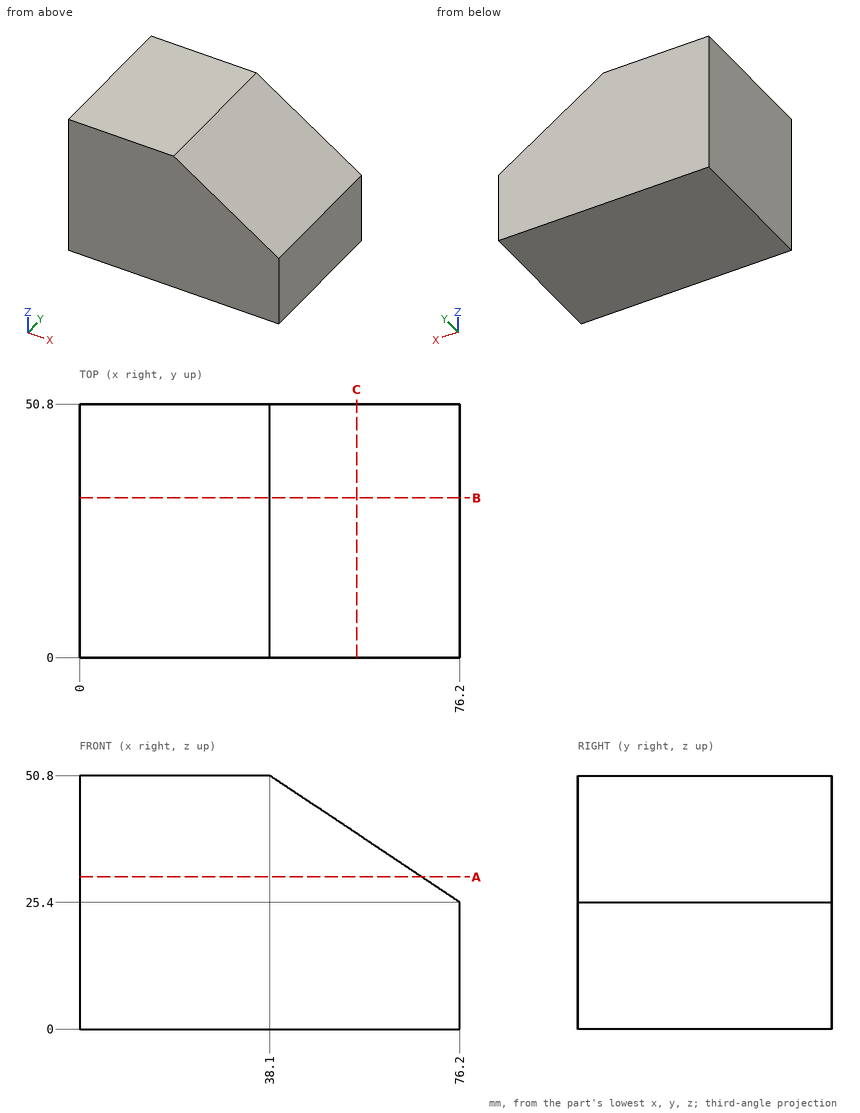
Job drawing, mm, ordinate dimensions from the low corner. One solid piece. Round coordinates to 2 decimals unless told otherwise and drop trailing zeros. Write each loop counter-clockwise with the first axis right and the second up, starting at its lowest first coordinate (ties: lowest second). Pieces come first, ordered by that corner, then holes. Notation, with made-up numbers: M 45,38.25 L 101,38.25 A10 cw 101,44.25 Z; hole C -19,29 d5. An arc over 180 degrees is marked long. Return JSON: item names as keys, results as strings. Group by question number.
(1) Pin check, flat tips, straight feed: pin 1 Ø3 at (x, z) = (65, 37) entering from +Y; pin 2 Ø5 at (y, z) = (9, 31.5) entering from +X. Stop position of each tip, or through.
(2) Saw through at A-A on z = 30.5. Write the cut outline in (x, y), then the cut area to 3 significant figures.
(3) Saw through at C-C on x = 55.5. Write the cut outline in (y, z), then the cut area to 3 significant figures.
(4) Saw through at B-B on y = 32. Write the cut outline in (x, z), then the cut area to 3 significant figures.
(5) Drill centre lines: probe 1 along Z at (x, y) = (54.5, 13); probe 2 along Z at (x, y) = (73.5, 25); probe 3 along X at (y, z) = (6, 27). Where is each one in solid material? Low to high.
Returned:
{
 "1": {"pin 1": "through", "pin 2": "x = 70.8"},
 "2": {"outline": "M 0,0 L 68.55,0 L 68.55,50.8 L 0,50.8 Z", "area": "3,480 mm²"},
 "3": {"outline": "M 0,0 L 50.8,0 L 50.8,39.2 L 0,39.2 Z", "area": "1,990 mm²"},
 "4": {"outline": "M 0,0 L 76.2,0 L 76.2,25.4 L 38.1,50.8 L 0,50.8 Z", "area": "3,390 mm²"},
 "5": {"probe 1": "0 to 39.87", "probe 2": "0 to 27.2", "probe 3": "0 to 73.8"}
}
